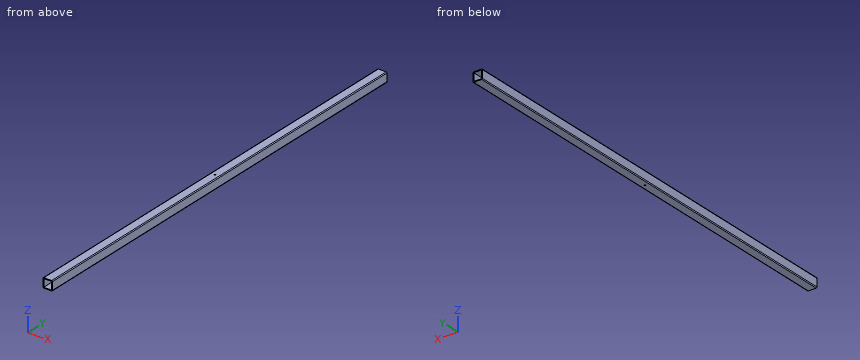
from build123d import *

# Parameters (mm, degrees)
F0_W     = 38.1
F0_H     = 38.1
F0_W_2   = 31.75
F0_H_2   = 31.75
F1_DEPTH = 1778
F2_R     = 3.175
F4_DEPTH = 38.101


with BuildPart() as f1:
    # F0 (on Front) → F1 (new body)
    with BuildSketch(Plane.XZ):
        Rectangle(F0_W, F0_H)
        Rectangle(F0_W_2, F0_H_2, mode=Mode.SUBTRACT)
    extrude(amount=F1_DEPTH)

    # F2
    f2_edges = [f1.edges().sort_by_distance(p)[0] for p in [
        (19.05, -889, 19.05),
        (19.05, -889, -19.05),
        (-19.05, -889, -19.05),
        (-19.05, -889, 19.05),
    ]]
    fillet(f2_edges, radius=F2_R)

    # F3 (on face) → F4 (cut, through all)
    with BuildSketch(Plane.XY.offset(19.05)):
        with BuildLine():
            ThreePointArc((0, -885.825), (-2.245064, -891.245064), (3.175, -889))
            ThreePointArc((3.175, -889), (2.245064, -886.754936), (0, -885.825))
        make_face()
    extrude(amount=-F4_DEPTH, mode=Mode.SUBTRACT)


solid = f1.part
The model under review builds one solid part; all positions refer to its coordinate system, in mm. Round coordinates to 2 decimals unless told otherwise and drop trailing zeros. Write each loop counter-clockwise with the first axis right and the second up, starting at its lowest first coordinate (ties: lowest second). Pieces come first, ordered by that corner, then holes. Notation, with made-up numbers: M 88.5,78.5 L 140.5,78.5 A24 cw 140.5,94.5 Z; hole C -33.5,8.25 d2. An arc over 180 degrees is marked long. Answer as CSV lines item,"result". Start each with the question number.
Q1. Wall thickness on line 1 along Z through (x, y) = (-7, -1062) (3 decimals); line 2 along X through (y, z) = (-889, -16) (3 decimals): over which ranges is each line inside the solid? List them lowest first.
Q2. Consider section B-B, the plane x = 10. Give the boundary of the cut face in (y, z) (3 decimals), then the cut area to 3 significant figures.
Q3. Consider section C-C, the plane y = -516. Give the boundary of the cut face in (x, z) (3 decimals).
Q4. Consider section A-A, the plane z = -2.5. Give the boundary of the cut face in (x, y) (3 decimals), then the cut area to 3 significant figures.
Q5. Clearance check with a flat-ended pin moving along its axis: P1, Ø10, axis at x = 0, y = -889, coming from the -Z side. State where the tip first meets the part, or that it passes through.
Result set:
1,line 1,"z = -19.05 to -15.875, 15.875 to 19.05"
1,line 2,"x = -19.048 to -3.175, 3.175 to 19.048"
2,outline,"M -1778,-19.05 L 0,-19.05 L 0,-15.875 L -1778,-15.875 Z; M -1778,15.875 L 0,15.875 L 0,19.05 L -1778,19.05 Z"
2,area,"11,300 mm²"
3,outline,"M -19.05,-15.875 A3.175 ccw -15.875,-19.05 L 15.875,-19.05 A3.175 ccw 19.05,-15.875 L 19.05,15.875 A3.175 ccw 15.875,19.05 L -15.875,19.05 A3.175 ccw -19.05,15.875 Z; hole M -15.875,-15.875 L 15.875,-15.875 L 15.875,15.875 L -15.875,15.875 Z"
4,outline,"M -19.05,-1778 L -15.875,-1778 L -15.875,0 L -19.05,0 Z; M 15.875,-1778 L 19.05,-1778 L 19.05,0 L 15.875,0 Z"
4,area,"11,300 mm²"
5,P1,"stops at z = -19.05"
